For this review, take the finished solid that the model builds, in its own axes (mm). Face numbers are marked on the shaded views. A direction names the side the tool comes from. Coordinates: 2 decimals unless noted, no trailing zeros. Order: outer loops, then holes, each group sorted by start corner. A loop starts at its lowest first (then second) coordinate and runs counter-clockwise, first axis right, second up. Notation, with made-up numbers: (73.25, 78.5) -> (78.25, 78.5) arc R28 cw to (78.25, 111.5) -> close; hole circle Ø11 at (63, 60.25). An arc over 180 degrees is marked (long way). Answer as a JSON object with one key per item and string values. Group by question number.
1) Draft analysis for pull direction X (two halves, no side actions). For the marked faces 6 and 7, state which applies: +X half, -X half, draft (parallel to the pull), parting line (faces both ways), or undercut.
2) For pin 1 (3 mm diameter, centred on x = -20.5, z = 1.5, fed in from +Y); pin 2 (10 mm diameter, centred on x = -6, y = 42, fed in from +Z); pin 3 (10 mm diameter, centred on x = 44, y = 16, fed in from -Z), all flat-tipped, find the tip position at first contact; note any pin that passes through.
3) Add section C-C, the plane z = -16. Write out the cut boundary in (x, y).
4) Add section B-B, the plane x = -30. Write out the cut boundary in (y, z), then the cut area to 3 significant figures.
5) Wall thickness on L1, parallel to Y at x = 68.9, z = -22.5; L2, parallel to Z at x = -57, y = 6; L3, parallel to Z at x = 30, y = 3.25: over which ranges is each line inside the solid? List them lowest first.
6) Machinability: for the marked faces 1, 2, 3, 4 and 5, which of the approach directions +Z, -Z, +X, -X, +Y, -Y give a long, thin tool a straight path to every point of the face, cutting with its end or side? Answer none if there is none.
7) Add section D-D, the plane x = -57.5. Write out the cut boundary in (y, z), then the cut area to 3 significant figures.
8) Add section A-A, the plane y = 45. Write out the cut boundary in (x, z).
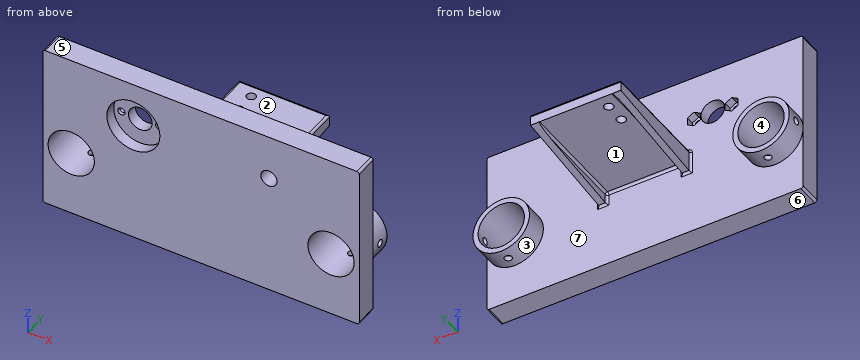
from build123d import *

# Parameters (mm, degrees)
SALIENTE_EXTRUIR1_DEPTH = 10
CROQUIS3_R              = 5.25
CROQUIS3_R_2            = 3.6
CROQUIS3_R_3            = 1.6
CORTAR_EXTRUIR1_DEPTH   = 11
CORTAR_EXTRUIR2_DEPTH   = 3.5
CROQUIS5_R              = 11.75
CORTAR_EXTRUIR3_DEPTH   = 5
CROQUIS8_W              = 90
CROQUIS8_H              = 29
SALIENTE_EXTRUIR2_DEPTH = 10
CROQUIS9_W              = 25
CROQUIS9_H              = 25
SALIENTE_EXTRUIR4_DEPTH = 10
CROQUIS13_R             = 12.5
SALIENTE_EXTRUIR5_DEPTH = 10
CROQUIS15_R             = 10.25
CORTAR_EXTRUIR5_DEPTH   = 20
CROQUIS16_R             = 1.6
CORTAR_EXTRUIR6_DEPTH   = 10
CROQUIS17_W             = 25
CROQUIS17_H             = 16.5
CROQUIS17_H_2           = 32.5
SALIENTE_EXTRUIR6_DEPTH = 10
CORTAR_EXTRUIR10_START  = 60
CROQUIS19_R             = 1.6
CORTAR_EXTRUIR10_DEPTH  = 11.0000001
SALIENTE_EXTRUIR7_DEPTH = 50
CROQUIS21_R             = 2
CORTAR_EXTRUIR11_DEPTH  = 40
CORTAR_EXTRUIR12_DEPTH  = 40
REDONDEO2_R             = 1
REDONDEO3_R             = 1


with BuildPart() as part:
    # Croquis1 → Saliente-Extruir1 (new body)
    with BuildSketch(Plane(origin=(0, 0, 0), x_dir=(1, 0, 0), z_dir=(0, 1, 0))):
        Polygon((-45, -22.5), (45, -22.5), (45, 22.5), (0, 22.5), (-45, 22.5), align=None)
    extrude(amount=SALIENTE_EXTRUIR1_DEPTH)

    # Croquis3 → Cortar-Extruir1 (cut, through all)
    with BuildSketch(Plane(origin=(0, 10, 0), x_dir=(1, 0, 0), z_dir=(0, 1, 0))):
        with Locations((-30, -2.5)):
            Circle(CROQUIS3_R)
        with Locations((30, -2.5)):
            Circle(CROQUIS3_R_2)
        with Locations((-38.375, -2.5)):
            Circle(CROQUIS3_R_3)
        with Locations((-21.625, -2.5)):
            Circle(CROQUIS3_R_3)
    extrude(amount=-CORTAR_EXTRUIR1_DEPTH, mode=Mode.SUBTRACT)

    # Croquis4 → Cortar-Extruir2 (cut)
    with BuildSketch(Plane(origin=(0, 10, 0), x_dir=(1, 0, 0), z_dir=(0, 1, 0))):
        Polygon((-38.375, 0.790896534), (-41.225, -0.854551733), (-41.225, -4.145448267), (-38.375, -5.790896534), (-35.525, -4.145448267), (-35.525, -0.854551733), align=None)
        Polygon((-21.625, 0.790896534), (-24.475, -0.854551733), (-24.475, -4.145448267), (-21.625, -5.790896534), (-18.775, -4.145448267), (-18.775, -0.854551733), align=None)
    extrude(amount=-CORTAR_EXTRUIR2_DEPTH, mode=Mode.SUBTRACT)

    # Croquis5 → Cortar-Extruir3 (cut)
    with BuildSketch(Plane.XZ):
        with Locations((-30, 2.5)):
            Circle(CROQUIS5_R)
    extrude(amount=-CORTAR_EXTRUIR3_DEPTH, mode=Mode.SUBTRACT)

    # Croquis8 → Saliente-Extruir2 (add)
    with BuildSketch(Plane(origin=(0, 10, 0), x_dir=(1, 0, 0), z_dir=(0, 1, 0))):
        with Locations((0, 37)):
            Rectangle(CROQUIS8_W, CROQUIS8_H)
    extrude(amount=-SALIENTE_EXTRUIR2_DEPTH)

    # Croquis9 → Saliente-Extruir4 (add)
    with BuildSketch(Plane(origin=(0, 0, 0), x_dir=(1, 0, 0), z_dir=(0, 1, 0))):
        with Locations((-57.5, 22.5)):
            Rectangle(CROQUIS9_W, CROQUIS9_H)
        with Locations((57.5, 22.5)):
            Rectangle(CROQUIS9_W, CROQUIS9_H)
    extrude(amount=SALIENTE_EXTRUIR4_DEPTH)

    # Croquis13 → Saliente-Extruir5 (add)
    with BuildSketch(Plane(origin=(0, 10, 0), x_dir=(1, 0, 0), z_dir=(0, 1, 0))):
        with Locations((-57.5, 22.5)):
            Circle(CROQUIS13_R)
        with Locations((57.5, 22.5)):
            Circle(CROQUIS13_R)
    extrude(amount=SALIENTE_EXTRUIR5_DEPTH)

    # Croquis15 → Cortar-Extruir5 (cut)
    with BuildSketch(Plane(origin=(0, 20, 0), x_dir=(1, 0, 0), z_dir=(0, 1, 0))):
        with Locations((-57.5, 22.5)):
            Circle(CROQUIS15_R)
        with Locations((57.5, 22.5)):
            Circle(CROQUIS15_R)
    extrude(amount=-CORTAR_EXTRUIR5_DEPTH, mode=Mode.SUBTRACT)

    # Croquis16 → Cortar-Extruir6 (cut)
    with BuildSketch(Plane(origin=(0, 0, -35), x_dir=(-1, 0, 0), z_dir=(0, 0, -1))):
        with Locations((-57.5, 15)):
            Circle(CROQUIS16_R)
        with Locations((57.5, 15)):
            Circle(CROQUIS16_R)
    extrude(amount=-CORTAR_EXTRUIR6_DEPTH, mode=Mode.SUBTRACT)

    # Croquis17 → Saliente-Extruir6 (add)
    with BuildSketch(Plane(origin=(0, 0, 0), x_dir=(1, 0, 0), z_dir=(0, 1, 0))):
        with Locations((57.5, 43.25)):
            Rectangle(CROQUIS17_W, CROQUIS17_H)
        with Locations((57.5, -6.25)):
            Rectangle(CROQUIS17_W, CROQUIS17_H_2)
        with Locations((-57.5, 43.25)):
            Rectangle(CROQUIS17_W, CROQUIS17_H)
        with Locations((-57.5, -6.25)):
            Rectangle(CROQUIS17_W, CROQUIS17_H_2)
    extrude(amount=SALIENTE_EXTRUIR6_DEPTH)

    # Croquis19 → Cortar-Extruir10 (cut, through all)
    with BuildSketch(Plane(origin=(0, 0, 0), x_dir=(0, 0, -1), z_dir=(1, 0, 0)).offset(CORTAR_EXTRUIR10_START)):
        with Locations((22.5, 15)):
            Circle(CROQUIS19_R)
    cortar_extruir10 = extrude(amount=CORTAR_EXTRUIR10_DEPTH, mode=Mode.SUBTRACT)

    # Simetría1: Cortar-Extruir10 across plane
    add(cortar_extruir10.mirror(Plane(origin=(0, 0, 0), x_dir=(0, 0, 1), z_dir=(1, 0, 0))), mode=Mode.SUBTRACT)

    # Croquis20 → Saliente-Extruir7 (add)
    with BuildSketch(Plane(origin=(0, 10, 0), x_dir=(1, 0, 0), z_dir=(0, 1, 0))):
        Polygon((-20, 22.5), (-17, 22.5), (-17, 17.5), (17, 17.5), (17, 22.5), (20, 22.5), (20, 12.5), (-20, 12.5), align=None)
    extrude(amount=SALIENTE_EXTRUIR7_DEPTH)

    # Croquis21 → Cortar-Extruir11 (cut, through all)
    with BuildSketch(Plane.XY.offset(-12.5)):
        with Locations((-11, 54)):
            Circle(CROQUIS21_R)
        with Locations((-11, 45)):
            Circle(CROQUIS21_R)
    extrude(amount=-CORTAR_EXTRUIR11_DEPTH, mode=Mode.SUBTRACT)

    # Croquis22 → Cortar-Extruir12 (cut)
    with BuildSketch(Plane(origin=(20, 0, 0), x_dir=(0, 0, -1), z_dir=(1, 0, 0))):
        Polygon((17.5, 60), (22.5, 10), (22.5, 60), align=None)
    extrude(amount=-CORTAR_EXTRUIR12_DEPTH, mode=Mode.SUBTRACT)

    # Redondeo2
    redondeo2_edges = [part.edges().sort_by_distance(p)[0] for p in [
        (-70, 5, -51.5),
        (-70, 5, 22.5),
        (70, 5, -51.5),
        (70, 5, 22.5),
    ]]
    fillet(redondeo2_edges, radius=REDONDEO2_R)

    # Redondeo3
    redondeo3_edges = [part.edges().sort_by_distance(p)[0] for p in [
        (-20, 10, -17.5),
        (0, 10, -12.5),
        (-20, 35, -12.5),
        (20, 10, -17.5),
        (20, 35, -12.5),
        (18.5, 10, -22.5),
        (17, 10, -20),
        (0, 10, -17.5),
        (17, 35, -17.5),
        (-17, 10, -20),
        (-17, 35, -17.5),
        (-18.5, 10, -22.5),
        (0, 60, -12.5),
    ]]
    fillet(redondeo3_edges, radius=REDONDEO3_R)


solid = part.part
Output values:
{
 "1": {"face 6": "draft", "face 7": "undercut"},
 "2": {"pin 1": "stops at y = 10", "pin 2": "stops at z = -12.5", "pin 3": "stops at z = -31.67"},
 "3": {"outline": "(-70, 0) -> (-65.43, 0) -> (-65.43, 20) -> (-68.18, 20) -> (-68.18, 10) -> (-70, 10) -> close; (-49.57, 0) -> (49.57, 0) -> (49.57, 20) -> (46.82, 20) -> (46.82, 10) -> (21, 10) arc R1 cw to (20, 11) -> (20, 60) -> (-20, 60) -> (-20, 11) arc R1 cw to (-21, 10) -> (-46.82, 10) -> (-46.82, 20) -> (-49.57, 20) -> close; (65.43, 0) -> (70, 0) -> (70, 10) -> (68.18, 10) -> (68.18, 20) -> (65.43, 20) -> close; hole circle Ø4 at (-11, 45); hole circle Ø4 at (-11, 54)"},
 "4": {"outline": "(0, -51.5) -> (10, -51.5) -> (10, -2.75) -> (5, -2.75) -> (5, -9.25) -> (0, -9.25) -> close; (0, 14.25) -> (5, 14.25) -> (5, 7.75) -> (10, 7.75) -> (10, 22.5) -> (0, 22.5) -> close", "area": "570 mm²"},
 "5": {"L1": "y = 0 to 13.4, 16.6 to 20", "L2": "z = -51.5 to -32.74, -12.26 to 22.5", "L3": "z = -51.5 to -1.1, 6.1 to 22.5"},
 "6": {"face 1": "-Z, +Y", "face 2": "+Z, +Y", "face 3": "+Y", "face 4": "+Y, -Y", "face 5": "+Z, +X, -X, +Y, -Y"},
 "7": {"outline": "(0, -51.5) -> (10, -51.5) -> (10, -35) -> (13.4, -35) -> (13.4, -32.75) -> (0, -32.75) -> close; (0, -12.25) -> (20, -12.25) -> (20, -10) -> (10, -10) -> (10, 22.5) -> (0, 22.5) -> close; (16.6, -35) -> (20, -35) -> (20, -32.75) -> (16.6, -32.75) -> close", "area": "573 mm²"},
 "8": {"outline": "(-20, -19) -> (-17, -19) -> (-17, -18.5) arc R1 cw to (-16, -17.5) -> (-13, -17.5) -> (-13, -12.5) -> (-19, -12.5) arc R1 ccw to (-20, -13.5) -> close; (-9, -17.5) -> (16, -17.5) arc R1 cw to (17, -18.5) -> (17, -19) -> (20, -19) -> (20, -13.5) arc R1 ccw to (19, -12.5) -> (-9, -12.5) -> close"}
}
